```python
from build123d import *

# Parameters (mm, degrees)
SKETCH1_W           = 416.08
SKETCH1_H           = 416.08
BOSS_EXTRUDE1_DEPTH = 3.175
SKETCH4_W           = 16.914306981
SKETCH4_H           = 31.258998707
SKETCH4_W_2         = 29.9
SKETCH4_H_2         = 64.9
SKETCH4_W_3         = 64.9
SKETCH4_H_3         = 29.9
SKETCH4_W_4         = 30
CUT_EXTRUDE3_DEPTH  = 4.175


with BuildPart() as part:
    # Sketch1 → Boss-Extrude1 (new body)
    with BuildSketch(Plane(origin=(0, 0, 0), x_dir=(1, 0, 0), z_dir=(0, 1, 0))):
        with Locations((208.04, 208.04)):
            Rectangle(SKETCH1_W, SKETCH1_H)
    extrude(amount=BOSS_EXTRUDE1_DEPTH)

    # Sketch4 → Cut-Extrude3 (cut, through all)
    with BuildSketch(Plane.XZ):
        with Locations((69.139038516, -270.834733378)):
            Rectangle(SKETCH4_W, SKETCH4_H)
        with Locations((346.940961485, -270.834733378)):
            Rectangle(SKETCH4_W, SKETCH4_H)
        with Locations((401.13, -32.45)):
            Rectangle(SKETCH4_W_2, SKETCH4_H_2)
        with Locations((190.54, -14.95)):
            Rectangle(SKETCH4_W_3, SKETCH4_H_3)
        with Locations((15, -32.45)):
            Rectangle(SKETCH4_W_4, SKETCH4_H_2)
        with Locations((14.95, -282.03)):
            Rectangle(SKETCH4_W_2, SKETCH4_H_2)
        with Locations((401.13, -282.03)):
            Rectangle(SKETCH4_W_2, SKETCH4_H_2)
    extrude(amount=-CUT_EXTRUDE3_DEPTH, mode=Mode.SUBTRACT)


solid = part.part
```
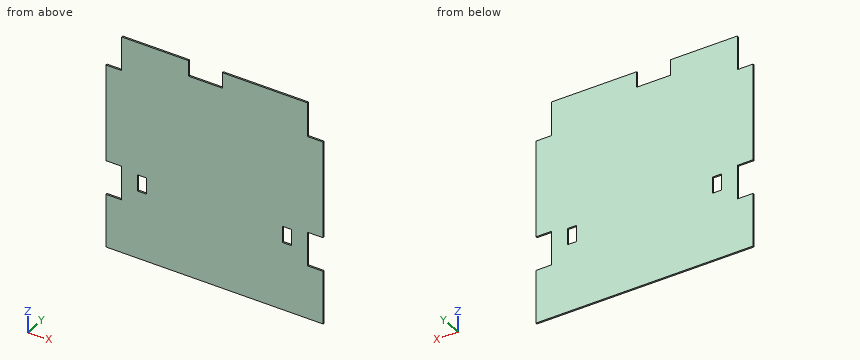
For this review, take the finished solid that the model builds, in its own axes (mm). Round coordinates to 2 decimals unless told otherwise and drop trailing zeros. Write each loop counter-clockwise with the first axis right and the second up, starting at its lowest first coordinate (ties: lowest second). Pieces come first, ordered by that corner, then holes. Notation, with made-up numbers: (70, 89.5) - (120, 89.5) arc R6 ccw to (120, 95.5) - close; hole circle Ø6 at (61, 79.25). An arc over 180 degrees is marked (long way). Answer as CSV lines item,"result". Start each with the question number.
(1) For line 1 (X direction, y = 1.8, z = -31); line 2 (X direction, y = 2.55, z = -309.5); line 3 (Z direction, x = 210, y = 0.2), list the stretches that pass through material, from the lowest coordinate up.
(2) For pin 1 (1.6 mm diameter, centred on y = 1, z = -269, fed in from -X); pin 2 (1 mm diameter, centred on y = 2, z = -290, fed in from +X); pin 3 (1.5 mm diameter, centred on x = 82, z = -120.5, fed in from -Y); pin 4 (1 mm diameter, centred on y = 1, z = -33, fed in from -X), all flat-tipped, find the tip position at first contact; note any pin that passes through.
(3) Add section C-C, the plane x = 194.5. State the section outline as (y, z) points (3 decimals), plus the area to 3 significant figures.
(4) Add section A-A, the plane z = -266.5. State the section outline as (x, y) points (3 decimals), plus the area to 3 significant figures.
(5) Add section B-B, the plane y = 1.65. State the section outline as (x, z) points.
From the geometry:
1,line 1,"x = 30 to 386.18"
1,line 2,"x = 29.9 to 386.18"
1,line 3,"z = -416.08 to -29.9"
2,pin 1,"stops at x = 29.9"
2,pin 2,"stops at x = 386.18"
2,pin 3,"stops at y = 0"
2,pin 4,"stops at x = 30"
3,outline,"(0, -416.08) - (3.175, -416.08) - (3.175, -29.9) - (0, -29.9) - close"
3,area,"1,230 mm²"
4,outline,"(29.9, 0) - (60.682, 0) - (60.682, 3.175) - (29.9, 3.175) - close; (77.596, 0) - (338.484, 0) - (338.484, 3.175) - (77.596, 3.175) - close; (355.398, 0) - (386.18, 0) - (386.18, 3.175) - (355.398, 3.175) - close"
4,area,"1,020 mm²"
5,outline,"(0, -416.08) - (416.08, -416.08) - (416.08, -314.48) - (386.18, -314.48) - (386.18, -249.58) - (416.08, -249.58) - (416.08, -64.9) - (386.18, -64.9) - (386.18, 0) - (222.99, 0) - (222.99, -29.9) - (158.09, -29.9) - (158.09, 0) - (30, 0) - (30, -64.9) - (0, -64.9) - (0, -249.58) - (29.9, -249.58) - (29.9, -314.48) - (0, -314.48) - close; hole (60.68, -286.46) - (77.6, -286.46) - (77.6, -255.21) - (60.68, -255.21) - close; hole (338.48, -286.46) - (355.4, -286.46) - (355.4, -255.21) - (338.48, -255.21) - close"
